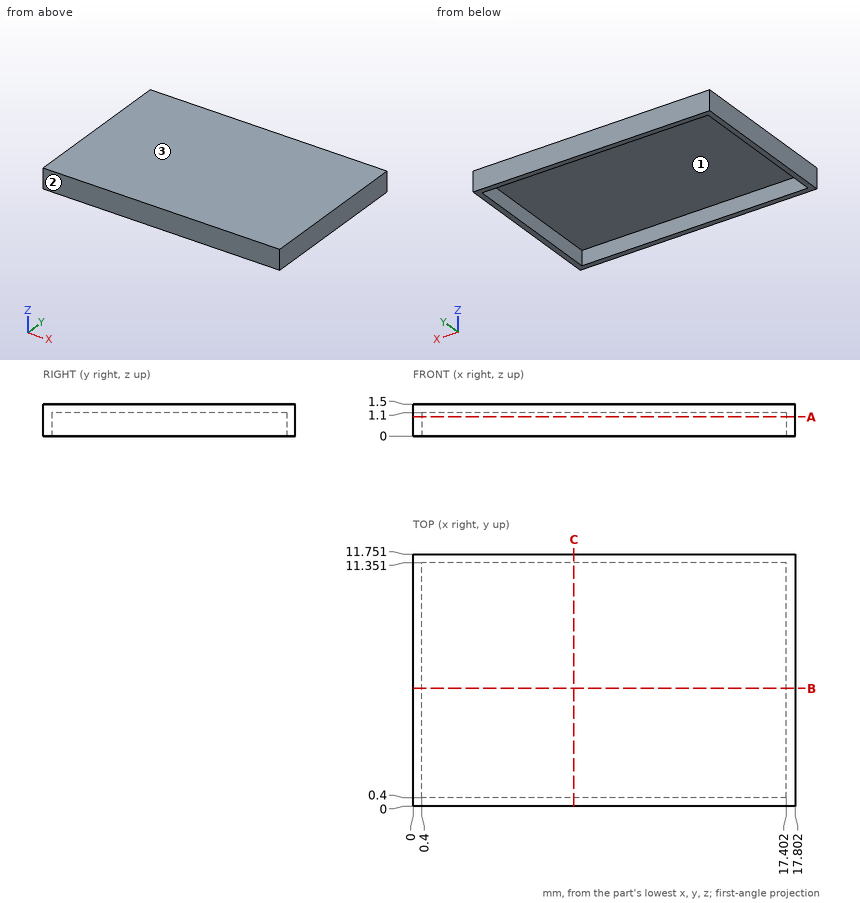
Print and shaded views of the part. All mm, measured from the part's lowest x, y and z. Coordinates: 2 decimals unless noted, no trailing zeros. Order: outer loops, then holes, each group sorted by start corner. A loop starts at its lowest first (then second) coordinate and runs counter-clockwise, first axis right, second up. Notation, with made-up numbers: (11, 33.25) -> (49, 33.25) arc R32 ccw to (49, 59.25) -> close; hole circle Ø7 at (48.5, 89.5). An arc over 180 degrees is marked (long way). Answer as a JSON object with one key per item and string values. Group by question number.
1) Drill centre lines: L1, parallel to Y at x = 7.5, z = 0.45; L2, parallel to X at y = 4.25, z = 0.9; L3, parallel to Z at x = 5.25, y = 2.5. Where is each one in solid material? Low to high.
2) Pull direction Y, two halves, no side cores. Call the marked faces 1, 2 and 3: +Y half, -Y half, draft (parallel to the pull), parting line (faces both ways), or undercut.
3) Cut at B-B, the plane y = 5.5. Write the cut outline in (x, z).
4) Cut at A-A, the plane z = 0.9. Write the cut outline in (x, y).
5) Cut at C-C, the plane x = 7.5. Write the cut outline in (y, z).
6) Flat gauge pin, fed straight in: pin 1 (3 mm diameter, centred on x = 9.5, y = 9, fed in from -Z). Where does the tip first touch, or does it go through?
Check values:
{
 "1": {"L1": "y = 0 to 0.4, 11.35 to 11.75", "L2": "x = 0 to 0.4, 17.4 to 17.8", "L3": "z = 1.1 to 1.5"},
 "2": {"face 1": "undercut", "face 2": "-Y half", "face 3": "draft"},
 "3": {"outline": "(0, 0) -> (0.4, 0) -> (0.4, 1.1) -> (17.4, 1.1) -> (17.4, 0) -> (17.8, 0) -> (17.8, 1.5) -> (0, 1.5) -> close"},
 "4": {"outline": "(0, 0) -> (17.8, 0) -> (17.8, 11.75) -> (0, 11.75) -> close; hole (0.4, 0.4) -> (17.4, 0.4) -> (17.4, 11.35) -> (0.4, 11.35) -> close"},
 "5": {"outline": "(0, 0) -> (0.4, 0) -> (0.4, 1.1) -> (11.35, 1.1) -> (11.35, 0) -> (11.75, 0) -> (11.75, 1.5) -> (0, 1.5) -> close"},
 "6": {"pin 1": "stops at z = 1.1"}
}
